Geometry check sheet. Reference: the model listing, model coordinates, mm. Face numbers are marked on the shaded views. A direction names the side the tool comes from. Round coordinates to 2 decimals unless told otherwise and drop trailing zeros. Order: outer loops, then holes, each group sorted by start corner. A loop starts at its lowest first (then second) coordinate and runs counter-clockwise, first axis right, second up.
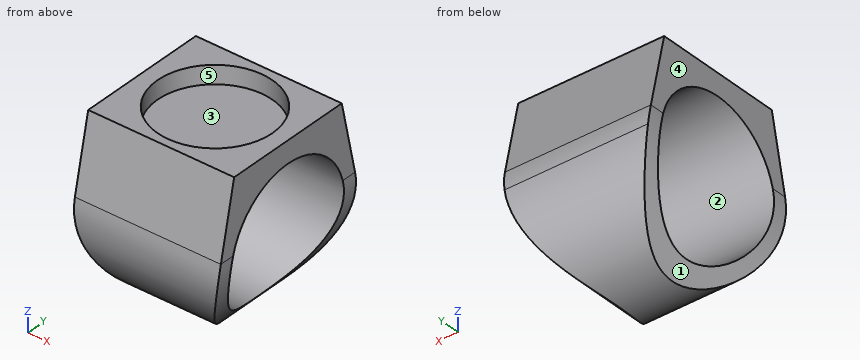
```python
from build123d import *

# Parameters (mm, degrees)
F0_R     = 9.5
F1_DEPTH = 10
F3_DEPTH = 15
F4_R     = 7.875
F5_DEPTH = 2.5


with BuildPart() as f1:
    # F0 (on Right) → F1 (new body, symmetric)
    with BuildSketch(Plane.YZ):
        with BuildLine():
            ThreePointArc((-11.225497, 2.497642), (-1.256341, -11.431168), (11.5, 0))
            ThreePointArc((11.5, 0), (11.431168, 1.256341), (11.225497, 2.497642))
            ThreePointArc((11.225497, 2.497642), (0, 11.5), (-11.225497, 2.497642))
        make_face()
        Circle(F0_R, mode=Mode.SUBTRACT)
        with BuildLine():
            ThreePointArc((-11.225497, 2.497642), (0, 11.5), (11.225497, 2.497642))
            Line((11.225497, 2.497642), (9, 12.5))
            Line((9, 12.5), (-9, 12.5))
            Line((-9, 12.5), (-11.225497, 2.497642))
        make_face()
    extrude(amount=F1_DEPTH, both=True)

    # F2 (on Front) → F3 (cut, symmetric)
    with BuildSketch(Plane.XZ):
        with BuildLine():
            Line((10, 12.5), (10, 2.5))
            ThreePointArc((10, 2.5), (8.02051, -5.885255), (2.5, -12.5))
            Line((2.5, -12.5), (-2.5, -12.5))
            ThreePointArc((-2.5, -12.5), (-8.02051, -5.885255), (-10, 2.5))
            Line((-10, 2.5), (-10, 12.5))
            Line((-10, 12.5), (-15, 12.5))
            Line((-15, 12.5), (-15, -17.5))
            Line((-15, -17.5), (15, -17.5))
            Line((15, -17.5), (15, 12.5))
            Line((15, 12.5), (10, 12.5))
        make_face()
    extrude(amount=F3_DEPTH, both=True, mode=Mode.SUBTRACT)

    # F4 (on face) → F5 (cut)
    with BuildSketch(Plane.XY.offset(12.5)):
        Circle(F4_R)
    extrude(amount=-F5_DEPTH, mode=Mode.SUBTRACT)


solid = f1.part
```
(1) Sectioned sample at A-A, the plane x = 0. Record the cut outline in (y, z) (1 decimal), and give its area (3 significant figures).
Returned:
outline: (-11.2, 2.5) arc R11.5 ccw (long way) to (11.5, 0) arc R11.5 ccw to (11.2, 2.5) - (9, 12.5) - (7.9, 12.5) - (7.9, 10) - (-7.9, 10) - (-7.9, 12.5) - (-9, 12.5) - close; hole circle Ø19 at (0, 0)
area: 144 mm2
(2) Sectioned sample at D-D, the plane x = 8.5. Record the cut outline in (y, z), and give its area (3 significant figures).
Returned:
outline: (-11.23, 2.5) arc R11.5 ccw to (-10.43, -4.85) - (-8.17, -4.85) arc R9.5 cw (long way) to (8.17, -4.85) - (10.43, -4.85) arc R11.5 ccw to (11.5, 0) arc R11.5 ccw to (11.23, 2.5) - (9, 12.5) - (-9, 12.5) - close
area: 138 mm2
(3) Depth check by flat-ended pin: P1, Ø1.5, axis at x = -3, z = 9.5, coming from the -Y side; P2, Ø9.5, axis at x = 0, y = 0, coming from the +Z side; P3, Ø10, axis at y = -3.5, z = -7, coming from the +X side. Enter the tip coordinate at first touch or a pass-through.
Returned:
P1: stops at y = -9.83
P2: stops at z = 10
P3: stops at x = 8.44
(4) Sectioned sample at B-B, the plane y = -2.25. Record the cut outline in (x, z), and give its area (3 significant figures).
Returned:
outline: (-10, 9.23) - (10, 9.23) - (10, 12.5) - (7.55, 12.5) - (7.55, 10) - (-7.55, 10) - (-7.55, 12.5) - (-10, 12.5) - close; (-5.88, -9.23) arc R18.75 ccw to (-3.97, -11.28) - (3.97, -11.28) arc R18.75 ccw to (5.88, -9.23) - close
area: 48.0 mm2
(5) Sectioned sample at C-C, the plane z = 2. Record the cut outline in (x, y), and give its area (3 significant figures).
Returned:
outline: (-9.99, -11.32) - (9.99, -11.32) - (9.99, -9.29) - (-9.99, -9.29) - close; (-9.99, 9.29) - (9.99, 9.29) - (9.99, 11.32) - (-9.99, 11.32) - close
area: 81.5 mm2
(6) Material ranges on line 1 (Y direction, x = -1.25, z = 0.25); line 2 (Z direction, x = 1.75, y = 0); line 3 (Z direction, x = -4.75, y = -5.25), recorded low to high.
Returned:
line 1: y = -11.5 to -9.5, 9.5 to 11.5
line 2: z = -11.5 to -9.5, 9.5 to 10
line 3: z = -10.23 to -7.92, 7.92 to 10
(7) Set-up check for the marked faces 4 and 5: record each of +Z, -Z, +X, -X, +Y, -Y from which the full face is reachable in a straight line by a thin tool's end or side.
Returned:
face 4: +Z, -Z, -X, +Y, -Y
face 5: +Z
(8) Draft check along Z on the marked faces 1, 2 and 3. Enter one of: released by +Z, released by -Z, zero draft, split by the parting line, or undercut.
Returned:
face 1: released by -Z
face 2: undercut
face 3: released by +Z
